from build123d import *

# Parameters (mm, degrees)
BOSS_EXTRU_1_DEPTH      = 5
ESQUISSE2_W             = 10
ESQUISSE2_H             = 10
ESQUISSE2_W_2           = 25
ESQUISSE2_H_2           = 6
BOSS_EXTRU_2_DEPTH      = 3
ESQUISSE3_R             = 2.8
ENL_V_MAT_EXTRU_3_DEPTH = 8.1


with BuildPart() as part:
    # Esquisse1 → Boss.-Extru.1 (new body)
    with BuildSketch(Plane.XY):
        Polygon((0, 0), (60, 0), (60, -10), (38.522739923, -19.314739888), (36.355716988, -24.967843196), (41.356924968, -33.188115427), (41.356924968, -53.188115427), (16.356924968, -53.188115427), (16.356924968, -43.188115427), (0, -10), align=None)
    extrude(amount=BOSS_EXTRU_1_DEPTH)

    # Esquisse2 → Boss.-Extru.2 (add)
    with BuildSketch(Plane(origin=(0, 0, 0), x_dir=(-1, 0, 0), z_dir=(0, 0, -1))):
        with Locations((-55, -5)):
            Rectangle(ESQUISSE2_W, ESQUISSE2_H)
        with Locations((-5, -5)):
            Rectangle(ESQUISSE2_W, ESQUISSE2_H)
        with Locations((-28.856924968, -43.188115427)):
            Rectangle(ESQUISSE2_W_2, ESQUISSE2_H_2)
    extrude(amount=BOSS_EXTRU_2_DEPTH)

    # Esquisse3 → Enlèv. mat.-Extru.3 (cut)
    with BuildSketch(Plane(origin=(0, 0, -3), x_dir=(-1, 0, 0), z_dir=(0, 0, -1))):
        with Locations((-56, -3.88)):
            Circle(ESQUISSE3_R)
        with Locations((-4, -3.88)):
            Circle(ESQUISSE3_R)
        with Locations((-28.856924968, -43.188115427)):
            Circle(ESQUISSE3_R)
    extrude(amount=-ENL_V_MAT_EXTRU_3_DEPTH, mode=Mode.SUBTRACT)


solid = part.part
Source: CAD feature listing. Evaluate the final solid. Frame: model axes, mm. A direction names the side the tool comes from. Round coordinates to 2 decimals unless told otherwise and drop trailing zeros. Loops run counter-clockwise (first coordinate to the right, second up) from the corner with the lowest first, then second, coordinate; pieces in that order, holes last. Notation, with made-up numbers: (-24, 3.25) - (-13, 3.25) arc R35 cw to (-13, 39.25) - close; hole circle Ø4 at (83.25, 17.25). An arc over 180 degrees is marked (long way). Write item = value, one per line. Start each with the question number.
(1) Section query C-C, the plane x = 56. Output: boundary loops of the cut face in (y, z).
(2) Section query D-D, the plane x = 4. Output: boundary loops of the cut face in (y, z), plus the area to 3 significant figures.
(3) Pin query (flat end, axial travel): pin 1 (12 mm diameter, centred on x = 43.5, y = -45, fed in from +Z); pin 2 (7.5 mm diameter, centred on x = 34, y = -50, fed in from -Z); pin 3 (1.5 mm diameter, centred on x = 6.5, z = -1.5, fed in from -Y); pin 4 (0.9 mm diameter, centred on x = 33.5, z = -1.5, fed in from -Y). Return the tip coordinate at first contact, or that it passes through.
(4) Set-up query: faces 1 (the face through (50, -5, -1)), 2 (the face through (5, -10, -1)), 3 (the face through (38.82, -29.02, 2.46)), 4 (the face through (41.357, -43, 2)). Return all of +Z, -Z, +X, -X, +Y, -Y with unobstructed straight access to the full face (end or side cutting, diameter ignored); none if empty.
(5) Pull-direction query (X, two-part tool) for faces 5 (the face through (10, -5, -1)), 6 (the face through (29, -50, 0)), 7 (the face through (16.357, -47, 2)); classes: +X half, -X half, draft (parallel to the pull), parting line (faces both ways), or undercut.
(6) Ray query, line 1 along X through (y, z) = (-6, -1.25); line 2 along Z through (x, y) = (32.5, -36.5); line 3 along Y through (x, z) = (56, 3.75). Return the intervals inside material, ascending. Write a range as from..to.
(7) Section query A-A, the plane y = -3.88. Output: boundary loops of the cut face in (x, z).
(8) Section query B-B, the plane z = 0.75. Output: boundary loops of the cut face in (x, y), plus the area to 3 significant figures.
Conclusion:
q1.outline = (-11.73, 0) - (-10, 0) - (-10, -3) - (-6.68, -3) - (-6.68, 5) - (-11.73, 5) - close; (-1.08, -3) - (0, -3) - (0, 5) - (-1.08, 5) - close
q2.outline = (-18.12, 0) - (-10, 0) - (-10, -3) - (-6.68, -3) - (-6.68, 5) - (-18.12, 5) - close; (-1.08, -3) - (0, -3) - (0, 5) - (-1.08, 5) - close
q2.area = 75.8 mm2
q3.pin_1 = 5
q3.pin_2 = 0
q3.pin_3 = -10
q3.pin_4 = -46.19
q4.face_1 = -Z, +Y, -Y
q4.face_2 = -Z, +X, -X, -Y
q4.face_3 = +Z, -Z, +X
q4.face_4 = +Z, -Z, +X, -Y
q5.face_5 = undercut
q5.face_6 = draft
q5.face_7 = -X half
q6.line_1 = 0..2.17, 5.83..10, 50..54.17, 57.83..60
q6.line_2 = 0..5
q6.line_3 = -11.73..-6.68, -1.08..0
q7.outline = (0, -3) - (1.2, -3) - (1.2, 5) - (0, 5) - close; (6.8, -3) - (10, -3) - (10, 0) - (50, 0) - (50, -3) - (53.2, -3) - (53.2, 5) - (6.8, 5) - close; (58.8, -3) - (60, -3) - (60, 5) - (58.8, 5) - close
q8.outline = (0, -10) - (16.36, -43.19) - (16.36, -53.19) - (41.36, -53.19) - (41.36, -33.19) - (36.36, -24.97) - (38.52, -19.31) - (60, -10) - (60, 0) - (0, 0) - close; hole circle Ø5.6 at (4, -3.88); hole circle Ø5.6 at (28.86, -43.19); hole circle Ø5.6 at (56, -3.88)
q8.area = 1,910 mm2
